from build123d import *

# Parameters (mm, degrees)
F1_DEPTH = 30
F2_R     = 4.4
F3_R     = 4.4
F4_DEPTH = 25
F5_R     = 2
F6_R     = 2


# Not quite as in the source:
# - a feature names something its author has since deleted; it is built from what else it names


with BuildPart() as f1:
    # F0 (on Front) → F1 (new body)
    with BuildSketch(Plane.XZ):
        Polygon((90, -1), (90, 1), (70, 1), (70, 49), (-70, 49), (-70, 1), (-90, 1), (-90, -1), (-68, -1), (-68, 47), (68, 47), (68, -1), align=None)
    extrude(amount=F1_DEPTH)

    # F2 (on face) + F3 (on face) → F4 (cut)
    with BuildSketch(Plane.XY.offset(1)):
        with Locations((-80, -15)):
            Circle(F2_R)
        with Locations((80, -15)):
            Circle(F2_R)
    with BuildSketch(Plane.XY.offset(49)):
        with Locations((-25, -15)):
            Circle(F3_R)
        with Locations((25, -15)):
            Circle(F3_R)
    extrude(amount=-F4_DEPTH, mode=Mode.SUBTRACT)

    # F5
    f5_edges = [f1.edges().sort_by_distance(p)[0] for p in [
        (-70, -15, 49),
        (70, -15, 49),
    ]]
    fillet(f5_edges, radius=F5_R)

    # F6
    f6_edges = [f1.edges().sort_by_distance(p)[0] for p in [
        (68, -15, -1),
        (-68, -15, -1),
    ]]
    fillet(f6_edges, radius=F6_R)


solid = f1.part
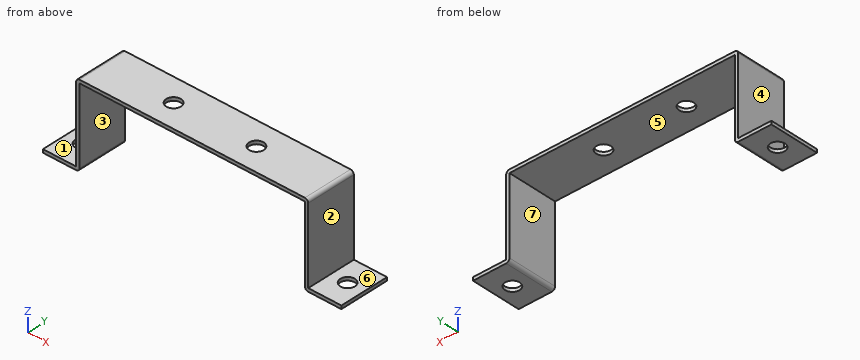
Part model, mm, in its own coordinate system. Face numbers are marked on the shaded views. A direction names the side the tool comes from. Round coordinates to 2 decimals unless told otherwise and drop trailing zeros. Order: outer loops, then holes, each group sorted by start corner. A loop starts at its lowest first (then second) coordinate and runs counter-clockwise, first axis right, second up. Notation, with made-up numbers: (29.5, 41.25) -> (69.5, 41.25) arc R24 ccw to (69.5, 62.25) -> close; hole circle Ø8 at (-13.75, 44). An arc over 180 degrees is marked (long way). Put each result on its own line as item: value.
Q1. Pin check, flat tips, straight feed: pin 1 Ø8 at (y, z) = (-11, 38.5) entering from +X; pin 2 Ø14 at (x, y) = (25, -15) entering from -Z; pin 3 Ø6 at (y, z) = (-15, 30.5) entering from -X. Stop position of each tip, or through.
From the geometry:
pin 1: stops at x = 70
pin 2: stops at z = 47
pin 3: stops at x = -70
Q2. Band-saw the part on A-A (y = -15). State how many separate pieces and enclosed holes the cut face has, and give its area (3 significant figures).
From the geometry:
separate pieces: 5
enclosed holes: 0
area: 478 mm2
Q3. Band-saw the part on D-D (x = 56). Give the cut face in (y, z), and give its area (3 significant figures).
From the geometry:
outline: (-30, 47) -> (0, 47) -> (0, 49) -> (-30, 49) -> close
area: 60.0 mm2
Q4. Band-saw the part on C-C (y = -23). Give the cut face in (x, z), and give its area (3 significant figures).
From the geometry:
outline: (-90, -1) -> (-70, -1) arc R2 ccw to (-68, 1) -> (-68, 47) -> (68, 47) -> (68, 1) arc R2 ccw to (70, -1) -> (90, -1) -> (90, 1) -> (70, 1) -> (70, 47) arc R2 ccw to (68, 49) -> (-68, 49) arc R2 ccw to (-70, 47) -> (-70, 1) -> (-90, 1) -> close
area: 549 mm2
Q5. Band-saw the part on B-B (x = 25). Give the cut face in (y, z), and give its area (3 significant figures).
From the geometry:
outline: (-30, 47) -> (-19.4, 47) -> (-19.4, 49) -> (-30, 49) -> close; (-10.6, 47) -> (0, 47) -> (0, 49) -> (-10.6, 49) -> close
area: 42.4 mm2
Q6. Tool access for the marked faces 1, 2 and 3: list every direction of +Z, -Z, +X, -X, +Y, -Y with a clear straight run to the whole face (end or side of a thin tool).
From the geometry:
face 1: +Z, -X, +Y, -Y
face 2: +Z, +X, +Y, -Y
face 3: -Z, +Y, -Y
Q7. Pull direction X, two halves, no side cores. Call the marked faces 4, 5, 6 and 7: pulls with the +X half, pulls with the -X half, needs draft (parallel to the pull), parting line crosses it, or undercut.
From the geometry:
face 4: pulls with the -X half
face 5: undercut
face 6: needs draft
face 7: undercut
Q8. Wall check: line 1 (X direction, y = -24, z = 8.5); line 2 (Y direction, x = -25, z = 47.4); line 3 (Z direction, x = 16.5, y = -20.25). Give the ranges that are in metal, low to high. Write a range as [from, to].
From the geometry:
line 1: x = [-70, -68], [68, 70]
line 2: y = [-30, -19.4], [-10.6, 0]
line 3: z = [47, 49]
